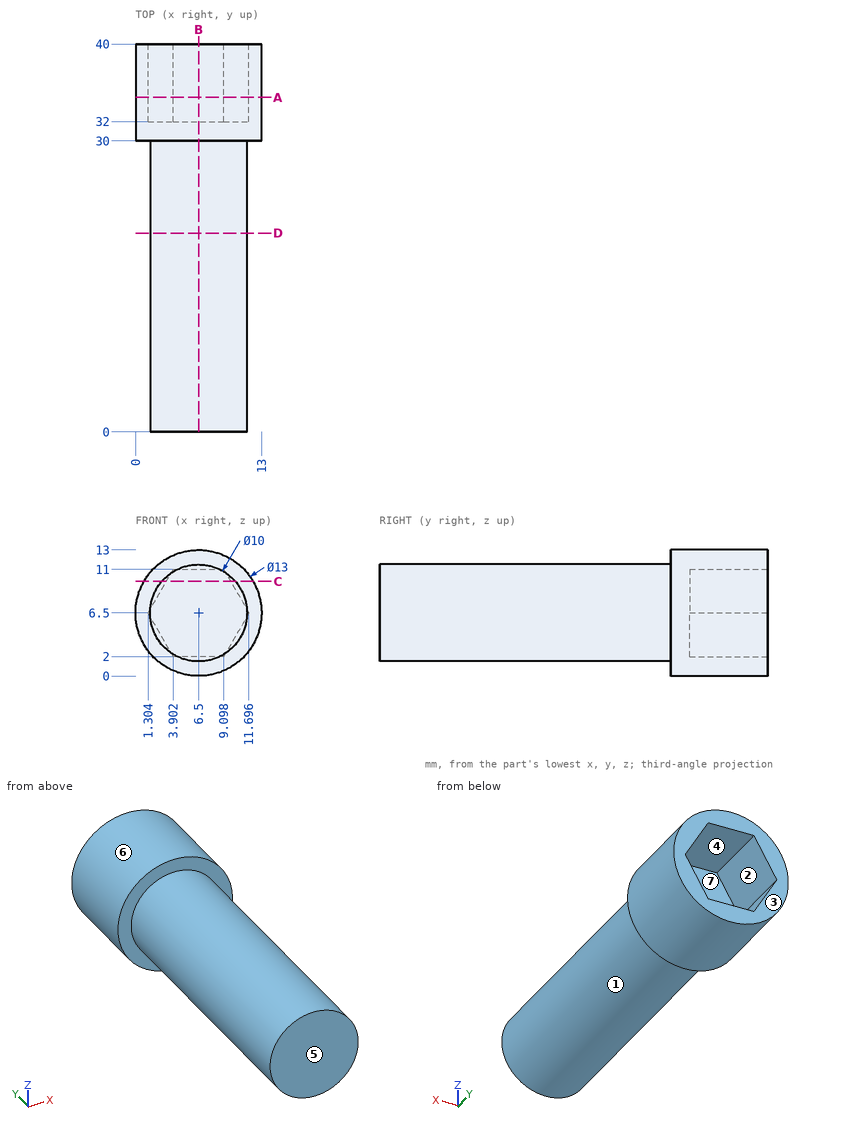
The drawing under review shows one solid part. Ordinate dimensions are in mm from its lowest x, y, z. A direction names the side the tool comes from. Coordinates: 2 decimals unless noted, no trailing zeros. Loops run counter-clockwise (first coordinate to the right, second up) from the corner with the lowest first, then second, coordinate; pieces in that order, holes last. Notation, with made-up numbers: (-3.75, 26) -> (45.25, 26) arc R25 cw to (45.25, 48) -> close; hole circle Ø2 at (-15.5, -21.75). An arc over 180 degrees is marked (long way). Answer as a JSON object with one key per item and string values.
Q1. Take a section at C-C on z = 9.75. Give the boundary of the cut face in (x, y), plus the area to 3 significant figures.
Answer block:
{"outline": "(0.87, 30) -> (2.7, 30) -> (2.7, 0) -> (10.3, 0) -> (10.3, 30) -> (12.13, 30) -> (12.13, 40) -> (9.82, 40) -> (9.82, 32) -> (3.18, 32) -> (3.18, 40) -> (0.87, 40) -> close", "area": "287 mm^2"}
Q2. To check wall thickness, follow L1, parallel to X at y = 34, z = 6.5; L2, parallel to Y at x = 4.5, z = 3.25; L3, parallel to Y at x = 3.5, z = 2. State the ranges of each line that lie inside material, in increasing order.
Answer block:
{"L1": "x = 0 to 1.3, 11.7 to 13", "L2": "y = 0 to 32", "L3": "y = 30 to 40"}
Q3. Take a section at A-A on y = 34.5. Give the boundary of the cut face in (x, z), plus the area to 3 significant figures.
Answer block:
{"outline": "circle Ø13 at (6.5, 6.5); hole (1.3, 6.5) -> (3.9, 2) -> (9.1, 2) -> (11.7, 6.5) -> (9.1, 11) -> (3.9, 11) -> close", "area": "62.6 mm^2"}
Q4. Clearance check with flat-ended pins moving along their axes: pin 1 Ø3 at (y, z) = (6, 11) entering from -X; pin 2 Ø1.6 at (x, y) = (8, 37) entering from -Z; pin 3 Ø2 at (x, y) = (8.5, 15.5) entering from -Z; pin 4 Ø7 at (x, z) = (5.5, 5) entering from +Y. State where each tip first meets the part, or that it passes through.
Answer block:
{"pin 1": "stops at x = 2.5", "pin 2": "stops at z = 0.04", "pin 3": "stops at z = 1.6", "pin 4": "stops at y = 40"}
Q5. Take a section at B-B on x = 6.5. Give the boundary of the cut face in (y, z).
Answer block:
{"outline": "(0, 1.5) -> (30, 1.5) -> (30, 0) -> (40, 0) -> (40, 2) -> (32, 2) -> (32, 11) -> (40, 11) -> (40, 13) -> (30, 13) -> (30, 11.5) -> (0, 11.5) -> close"}
Q6. The part is to be moulded in two halves that separate along X. For the marked faces 4, 5, 6 and 7, say which applies: +X half, -X half, draft (parallel to the pull), parting line (faces both ways), or undercut.
Answer block:
{"face 4": "undercut", "face 5": "draft", "face 6": "parting line", "face 7": "undercut"}
Q7. Tool access review of the marked faces 1, 2 and 3: name each direction out of +Z, -Z, +X, -X, +Y, -Y from which nothing blocks a thin tool from reaching the whole face with its end or side.
Answer block:
{"face 1": "-Y", "face 2": "+Y", "face 3": "+Z, -Z, +X, -X, +Y"}
Q8. Take a section at D-D on y = 20.5. Give the boundary of the cut face in (x, z).
Answer block:
{"outline": "circle Ø10 at (6.5, 6.5)"}
